For this review, take the finished solid that the model builds, in its own axes (mm). A direction names the side the tool comes from. Give positions to 0.01 mm unless a question says otherwise; leave off trailing zeros. Order: outer loops, then holes, each group sorted by start corner. A loop starts at its lowest first (then second) coordinate and runs counter-clockwise, first axis right, second up. Notation, with made-up numbers: (88, 11) - (114, 11) arc R21 cw to (114, 41) - close; hole circle Ø5 at (70, 41.5). An arc over 180 degrees is marked (long way). Answer as a JSON object with one key per item and string values. Group by question number.
from build123d import *

# Parameters (mm, degrees)
BOSS_EXTRUDE1_DEPTH = 9.5
SKETCH2_R           = 2
BOSS_EXTRUDE2_DEPTH = 19.5
SKETCH7_W           = 10
SKETCH7_H           = 5
CUT_EXTRUDE3_DEPTH  = 31.276334221
SKETCH5_R           = 3.302
SKETCH5_R_2         = 2.413
CUT_EXTRUDE2_DEPTH  = 3.5
FILLET3_R           = 10
FILLET1_R           = 1
FILLET2_R           = 1
SKETCH9_W           = 8
SKETCH9_H           = 8
CUT_EXTRUDE5_DEPTH  = 6.532330181
CHAMFER1_SIZE       = 3
CHAMFER1_SIZE_2     = 2.938727652


# Some blends are built 0.0001 mm under size
with BuildPart() as part:
    # Sketch1 → Boss-Extrude1 (new, symmetric)
    with BuildSketch(Plane.XY):
        with BuildLine():
            Line((0, 3.561668795), (-21, 17))
            Line((-21, 17), (-21.115416888, 3.14407423))
            Line((-21.115416888, 3.14407423), (-12.675875805, -1.822682799))
            Line((-12.675875805, -1.822682799), (-10.139894754, 2.486470263))
            Line((-10.139894754, 2.486470263), (-1.52158863, -2.585491837))
            ThreePointArc((-1.52158863, -2.585491837), (-0.972654449, -2.837947026), (-0.384266987, -2.975288034))
            Line((-0.384266987, -2.975288034), (7.549834435, -4))
            ThreePointArc((7.549834435, -4), (11.207454879, -1.17909917), (8.386554049, 2.478521273))
            Line((8.386554049, 2.478521273), (0, 3.561668795))
        make_face()
    extrude(amount=BOSS_EXTRUDE1_DEPTH, both=True)

    # Sketch2 → Boss-Extrude2 (add, symmetric)
    with BuildSketch(Plane.XY):
        with Locations(Location((0, 0, 0), (0, 0, 180))):
            Circle(SKETCH2_R)
    extrude(amount=BOSS_EXTRUDE2_DEPTH, both=True)

    # Sketch7 → Cut-Extrude3 (cut, through all)
    with BuildSketch(Plane(origin=(-8.618306124, 5.071962101, 0), x_dir=(0, 0, -1), z_dir=(0.8618306124209184, -0.5071962100550289, 0))):
        with Locations((0, -5.5)):
            Rectangle(SKETCH7_W, SKETCH7_H)
    extrude(amount=-CUT_EXTRUDE3_DEPTH, mode=Mode.SUBTRACT)

    # Sketch5 → Cut-Extrude2 (cut)
    with BuildSketch(Plane(origin=(-1.52158863, -2.585491837, 0), x_dir=(0.8618306124209184, -0.5071962100550289, 0), z_dir=(-0.5071962100550289, -0.8618306124209184, 0))):
        with Locations((-16.27, 0)):
            Circle(SKETCH5_R)
        with Locations((-16.27, 0)):
            Circle(SKETCH5_R_2, mode=Mode.SUBTRACT)
    extrude(amount=-CUT_EXTRUDE2_DEPTH, mode=Mode.SUBTRACT)

    # Fillet3
    # the kernel refuses this fillet: 10 mm, written as the material it takes off along each edge
    with BuildSketch(Plane(origin=(-12.675875805, -1.822682799, -31.150635095), x_dir=(-0.8618306124209182, 0.507196210055029, 0), z_dir=(0, 0, 1)), Plane(origin=(-12.675875805, -1.822682799, -16.650635095), x_dir=(-0.8618306124209182, 0.507196210055029, 0), z_dir=(0, 0, 1))) as fillet3_piece_1:
        with BuildLine():
            CenterArc((8.660254038, -10), FILLET3_R, 90, 60)
            Line((0, -5), (0, 0))
            Line((0, 0), (8.660254038, 0))
        make_face()
    extrude(amount=47.801270189, mode=Mode.SUBTRACT)

    # Fillet1
    fillet1_edges = [part.edges().sort_by_distance(p)[0] for p in [
        (-18.389337376, 7.341352386, 0),
        (-17.623169962, 6.890454955, 0),
    ]]
    fillet(fillet1_edges, radius=FILLET1_R)

    # Fillet2
    fillet2_edges = [part.edges().sort_by_distance(p)[0] for p in [
        (-0.972654449, -2.837947026, -9.5),
        (-5.830741692, -0.049510787, -9.5),
        (-10.5, 10.280834397, -9.5),
        (4.193277024, 3.020095034, -9.5),
        (0, 3.561668795, 0),
        (-5.830741692, -0.049510787, 9.5),
        (-0.972654449, -2.837947026, 9.5),
        (3.582783724, -3.487644017, 9.5),
        (11.207454879, -1.17909917, 9.5),
        (4.193277024, 3.020095034, 9.5),
        (-10.5, 10.280834397, 9.5),
        (11.207454879, -1.17909917, -9.5),
        (3.582783724, -3.487644017, -9.5),
    ]]
    fillet(fillet2_edges, radius=FILLET2_R - 0.0001)  # a hair under: the kernel refuses the full size

    # Sketch9 → Cut-Extrude5 (cut)
    with BuildSketch(Plane(origin=(0.452452626, 3.50323324, 0), x_dir=(0.9917626778378904, -0.12808899581079106, 0), z_dir=(0.12808899581079106, 0.9917626778378904, 0))):
        with Locations((7.266165091, 0)):
            Rectangle(SKETCH9_W, SKETCH9_H)
    extrude(amount=-CUT_EXTRUDE5_DEPTH, mode=Mode.SUBTRACT)

    # Chamfer1
    # the kernel refuses this chamfer: 5.196152423, 3.337326817, 3, 2.938727652 mm, written as the material it takes off along each edge
    with BuildSketch(Plane(origin=(-21, 17, -16.154510493), x_dir=(0.8423017896549276, -0.5390062106730368, 0), z_dir=(0, 0, 1))) as chamfer1_piece_1:
        Polygon((CHAMFER1_SIZE, 0), (CHAMFER1_SIZE_2 * 0.531971562398, -CHAMFER1_SIZE_2 * 0.846762219836), (0, 0), align=None)
    extrude(amount=32.309020987, mode=Mode.SUBTRACT)


solid = part.part
1) For faces 1 (the face through (-17.254, 9.264, 0.145)), 2 (the face through (-15.53, 5.66, 0.02)), 3 (the face through (3.28, -0.11, 0.06)), list the 3-axis set-ups (+Z, -Z, +X, -X, +Y, -Y) from which the entire face can be reached by the end or side of a thin tool; tool diameter is ignored.
2) For pin 1 (5 mm diameter, centred on x = 0.5, y = 7, fed in from -Z); pin 2 (3.5 mm diameter, centred on x = 5, y = 1, fed in from -Z); pin 3 (1 mm diameter, centred on x = -15.5, y = 7.5, fed in from +Z); pin 4 (10 mm diameter, centred on x = 8, z = 10.5, fed in from -Y), all flat-tipped, find the tip position at first contact; note any pin that passes through.
3) Mouldability with a two-part tool opening along X and no side actions: class faces 4 (the face through (-17, 4, 5)), 5 (the face through (-5.626, 0.161, 9.199)), 6 (the face through (0, 2, 15)), 7 (the face through (2.646, -3.367, 0.119)) as released by +X, released by -X, zero draft, split by the parting line, or undercut.
4) Consider section A-A (z = 15). Give the boundary of the cut face in (x, y).
5) For line 1 (Z direction, x = -2.5, y = 2.25); line 2 (Y direction, x = -3.5, z = 8.5); line 3 (X direction, y = 1.5, z = -0.5), list the stretches that pass through material, from the lowest coordinate up.
Result set:
{
 "1": {"face 1": "none", "face 2": "-X, -Y", "face 3": "+X, -Y"},
 "2": {"pin 1": "passes through", "pin 2": "stops at z = -9.5", "pin 3": "stops at z = 9.5", "pin 4": "stops at y = -4.03"},
 "3": {"face 4": "zero draft", "face 5": "undercut", "face 6": "split by the parting line", "face 7": "released by -X"},
 "4": {"outline": "circle Ø4 at (0, 0)"},
 "5": {"line 1": "z = -9.5 to 9.5", "line 2": "y = -1.42 to 5.8", "line 3": "x = -8.46 to 3.49"}
}
